```python
from build123d import *

# Parameters (mm, degrees)
SKETCH2_OUTSIDE_W   = 22.314
SKETCH2_OUTSIDE_H   = 22.314
SKETCH2_OUTSIDE_W_2 = 13
SKETCH2_OUTSIDE_H_2 = 17
CUT_EXTRUDE1_DEPTH  = 7
SKETCH3_R           = 5
BOSS_EXTRUDE1_DEPTH = 3
FILLET1_R           = 0.2


with BuildPart() as part:
    # Sketch1 → Revolve1 (revolve)
    with BuildSketch(Plane.XY, mode=Mode.PRIVATE) as revolve1_sk:
        with BuildLine():
            Line((0, 5.5), (-16, 5.5))
            Line((-16, 5.5), (-16, 6))
            Line((-16, 6), (-15.5, 6))
            ThreePointArc((-15.5, 6), (-14.439339828, 6.439339828), (-14, 7.5))
            Line((-14, 7.5), (0, 7.5))
            Line((0, 7.5), (0, 5.5))
        make_face()
    revolve(revolve1_sk.sketch.rotate(Axis((0, 0, 0), (-1, 0, 0)), 90), axis=Axis((0, 0, 0), (-1, 0, 0)))

    # Sketch2 outside → Cut-Extrude1 (cut)
    with BuildSketch(Plane(origin=(0, 0, 0), x_dir=(0, 0, -1), z_dir=(1, 0, 0))):
        Rectangle(SKETCH2_OUTSIDE_W, SKETCH2_OUTSIDE_H)
        Rectangle(SKETCH2_OUTSIDE_W_2, SKETCH2_OUTSIDE_H_2, mode=Mode.SUBTRACT)
    extrude(amount=-CUT_EXTRUDE1_DEPTH, mode=Mode.SUBTRACT)

    # Sketch3 → Boss-Extrude1 (add)
    with BuildSketch(Plane(origin=(0, 0, 0), x_dir=(0, 0, -1), z_dir=(1, 0, 0))):
        Polygon((9.814954576, 0), (4.907477288, 8.5), (-4.907477288, 8.5), (-9.814954576, 0), (-4.907477288, -8.5), (4.907477288, -8.5), align=None)
        Circle(SKETCH3_R, mode=Mode.SUBTRACT)
    extrude(amount=BOSS_EXTRUDE1_DEPTH)

    # Fillet1
    fillet1_edges = [part.edges().sort_by_distance(p)[0] for p in [
        (1.5, -8.5, -4.907477288),
        (1.5, 0, -9.814954576),
        (1.5, 8.5, -4.907477288),
        (1.5, 8.5, 4.907477288),
        (1.5, 0, 9.814954576),
        (1.5, -8.5, 4.907477288),
    ]]
    fillet(fillet1_edges, radius=FILLET1_R)


solid = part.part
```
Design review of the part built by this model. Coordinates are the model's own, in mm. A direction names the side the tool comes from. Give positions to 0.01 mm unless a question says otherwise; leave off trailing zeros. Loops run counter-clockwise (first coordinate to the right, second up) from the corner with the lowest first, then second, coordinate; pieces in that order, holes last. Notation, with made-up numbers: (48.25, -18) -> (57.25, -18) arc R13 cw to (57.25, -13) -> close; hole circle Ø9 at (-6.5, -6.5). An arc over 180 degrees is marked (long way). One line per item, written item: value.
Q1. We need section B-B on x = 1.75. Give the boundary of the cut face in (y, z), and give its area (3 significant figures).
Numbers:
outline: (-8.5, -4.79) arc R0.2 ccw to (-8.4, -4.97) -> (-0.1, -9.76) arc R0.2 ccw to (0.1, -9.76) -> (8.4, -4.97) arc R0.2 ccw to (8.5, -4.79) -> (8.5, 4.79) arc R0.2 ccw to (8.4, 4.97) -> (0.1, 9.76) arc R0.2 ccw to (-0.1, 9.76) -> (-8.4, 4.97) arc R0.2 ccw to (-8.5, 4.79) -> close; hole circle Ø10 at (0, 0)
area: 172 mm^2
Q2. Draft analysis for pull direction Z (two halves, no side actions). For faces 4 (the flat face through (1.479, 4.308, 7.328)), 5 (the flat face through (0, -4.9, -1.6)), 6 (the flat face through (-3, 0, -6.5)), state which applies: pulls with the +Z half, pulls with the -Z half, needs draft (parallel to the pull), parting line crosses it, or undercut.
Numbers:
face 4: pulls with the +Z half
face 5: undercut
face 6: pulls with the -Z half
Q3. For pin 1 Ø5.5 at (x, y) = (-5, 1) entering from +Z; pin 2 Ø3 at (x, z) = (-11, -7.5) entering from +Y; pin 3 Ø9 at (y, z) = (0, 0) entering from -X; pin 4 Ø3 at (x, y) = (-10.5, 3.5) entering from -Z, all flat-tipped, find the tip position at first contact; note any pin that passes through.
Numbers:
pin 1: stops at z = 7.5
pin 2: stops at y = 4.5
pin 3: passes through
pin 4: stops at z = -7.23
Q4. We need section C-C on x = -13.5. Give the boundary of the cut face in (y, z).
Numbers:
outline: circle Ø15 at (0, 0); hole circle Ø11 at (0, 0)
Q5. Machinability: for faces 1 (the flat face through (0, 0, 7)), 2 (the cylindrical face through (-8.11, 5.37, 1.19)), 3 (the flat face through (-3, 0, 6.5)), which of the approach directions +Z, -Z, +X, -X, +Y, -Y give a long, thin tool a straight path to every point of the face, cutting with its end or side? Answer none if there is none.
Numbers:
face 1: none
face 2: -X
face 3: +Z, +Y, -Y
Q6. For L1, parallel to Y at x = -9.5, z = 0; L2, parallel to Y at x = -2.5, z = -2; L3, parallel to Z at x = -0.75, y = 1, list the stretches that pass through material, from the lowest coordinate up.
Numbers:
L1: y = -7.5 to -5.5, 5.5 to 7.5
L2: y = -7.23 to -5.12, 5.12 to 7.23
L3: z = -6.5 to -5.41, 5.41 to 6.5
Q7. We need section A-A on z = 0. Give the boundary of the cut face in (x, y), and give its area (3 significant figures).
Numbers:
outline: (-16, -6) -> (-15.5, -6) arc R1.5 cw to (-14, -7.5) -> (0, -7.5) -> (0, -8.5) -> (3, -8.5) -> (3, -5) -> (0, -5) -> (0, -5.5) -> (-16, -5.5) -> close; (-16, 5.5) -> (0, 5.5) -> (0, 5) -> (3, 5) -> (3, 8.5) -> (0, 8.5) -> (0, 7.5) -> (-14, 7.5) arc R1.5 cw to (-15.5, 6) -> (-16, 6) -> close
area: 80.0 mm^2
